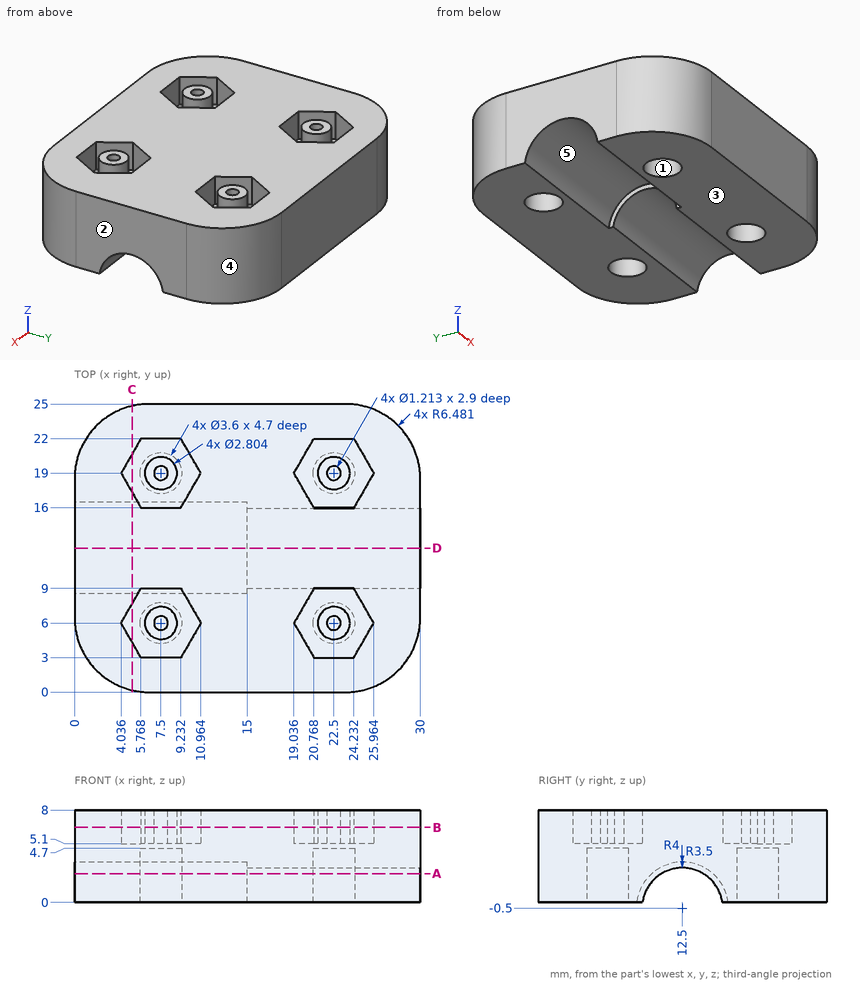
Job drawing, mm, ordinate dimensions from the low corner. One solid piece. A direction names the side the tool comes from. Give positions to 0.01 mm unless a question says otherwise; leave off trailing zeros. Order: outer loops, then holes, each group sorted by start corner. A loop starts at its lowest first (then second) coordinate and runs counter-clockwise, first axis right, second up. Notation, with made-up numbers: M 58.5,82.5 L 81.5,82.5 A24 ccw 81.5,119.5 Z; hole C 73,84.25 d4. An arc over 180 degrees is marked long. Put each result on its own line as item: value. Start each with the question number.
(1) Pin check, flat tips, straight feed: pin 1 Ø1 at (x, z) = (5, 4.5) entering from +Y (1 decimal); pin 2 Ø1.9 at (x, y) = (7.5, 19) entering from +Z; pin 3 Ø0.6 at (x, y) = (7.5, 19) entering from +Z; pin 4 Ø2 at (x, y) = (22.5, 6) entering from -Z. Stop position of each tip, or through.
(2) Band-saw the part on D-D on y = 12.5. Give the cut face in (x, z).
(3) Band-saw the part on B-B on z = 6.5. Count the separate pieces of the cut face and the enclosed holes in it.
(4) Band-saw the part on C-C on x = 5. Give the cut face in (y, z), then the cut area to 3 significant figures.
(5) Pull direction Y, two halves, no side cores. Call the marked faces 3, 4 and 5: released by +Y, released by -Y, zero draft, split by the parting line, or undercut.
(6) Band-saw the part on A-A on z = 2.5. Give the cut face in (x, y) (1 decimal).
(7) Drill centre lines: L1, parallel to X at y = 4.75, z = 7 (1 decimal); L2, parallel to Y at x = 22.5, z = 2.15 (1 decimal); L3, parallel to X at y = 6, z = 3.55. Where is each one in solid material? Low to high. Write a range as [from, to].
(8) Tool access for the marked faces 1 and 2: list every direction of +Z, -Z, +X, -X, +Y, -Y with a clear straight run to the whole face (end or side of a thin tool).
Results below:
1. pin 1: stops at y = 24.9
1. pin 2: stops at z = 8
1. pin 3: stops at z = 5.1
1. pin 4: stops at z = 4.7
2. outline: M 0,3.5 L 15,3.5 L 15,3 L 30,3 L 30,8 L 0,8 Z
3. separate pieces: 5
3. enclosed holes: 8
4. outline: M 0.17,0 L 8.53,0 A4 cw 16.47,0 L 24.83,0 L 24.83,8 L 20.67,8 L 20.67,5.1 L 17.33,5.1 L 17.33,8 L 7.67,8 L 7.67,5.1 L 4.33,5.1 L 4.33,8 L 0.17,8 Z
4. area: 157 mm2
5. face 3: zero draft
5. face 4: released by +Y
5. face 5: undercut
6. outline: M 0,6.5 A6.5 ccw 6.5,0 L 23.5,0 A6.5 ccw 30,6.5 L 30,10.7 L 15,10.7 L 15,9.9 L 0,9.9 Z; M 0,15.1 L 15,15.1 L 15,14.3 L 30,14.3 L 30,18.5 A6.5 ccw 23.5,25 L 6.5,25 A6.5 ccw 0,18.5 Z; hole C 7.5,6 d3.6; hole C 7.5,19 d3.6; hole C 22.5,6 d3.6; hole C 22.5,19 d3.6
7. L1: x = [0.2, 4.8], [6.9, 8.1], [10.2, 19.8], [21.9, 23.1], [25.2, 29.8]
7. L2: y = [0, 4.2], [7.8, 10.2], [14.8, 17.2], [20.8, 25]
7. L3: x = [0.02, 5.7], [9.3, 20.7], [24.3, 29.98]
8. face 1: -Z
8. face 2: +Z, -Z, +X, +Y, -Y
